Geometry check sheet. Reference: drawing and pictorial views, mm from the part's lowest x, y, z. A direction names the side the tool comes from. Round coordinates to 2 decimals unless told otherwise and drop trailing zeros. Write each loop counter-clockwise with the first axis right and the second up, starting at its lowest first coordinate (ties: lowest second). Pieces come first, ordered by that corner, then holes. Notation, with made-up numbers: (57.25, -2.5) -> (95.25, -2.5) arc R34 cw to (95.25, 30.5) -> close; hole circle Ø1 at (-16, -35.75). An arc over 180 degrees is marked (long way). Answer as a JSON object with one key per item and string values. Group by question number.
(1) Gauge pin test, flat ends, axial feed: pin 1 Ø4 at (x, z) = (964, 54) entering from -Y; pin 2 Ø8 at (x, y) = (710, 92.5) entering from +Z. Record the tip position at first contact, or that the pin passes through.
(2) Sectioned sample at A-A on z = 294.5. Record the cut outline in (x, y), and give its area (3 significant figures).
(3) Sectioned sample at B-B on x = 579. Record the cut outline in (y, z).
(4) Scan lines: L1, parallel to Y at x = 508, z = 308; L2, parallel to X at y = 81.5, z = 136.5. Record each from-to range of solid material in increasing order. Write a range as from..to.
(5) Sectioned sample at C-C on y = 43. Record the cut outline in (x, z), and give its area (3 significant figures).
(6) Set-up check for the marked faces 1 and 2: record each of +Z, -Z, +X, -X, +Y, -Y from which the full face is reachable in a straight line by a thin tool's end or side.
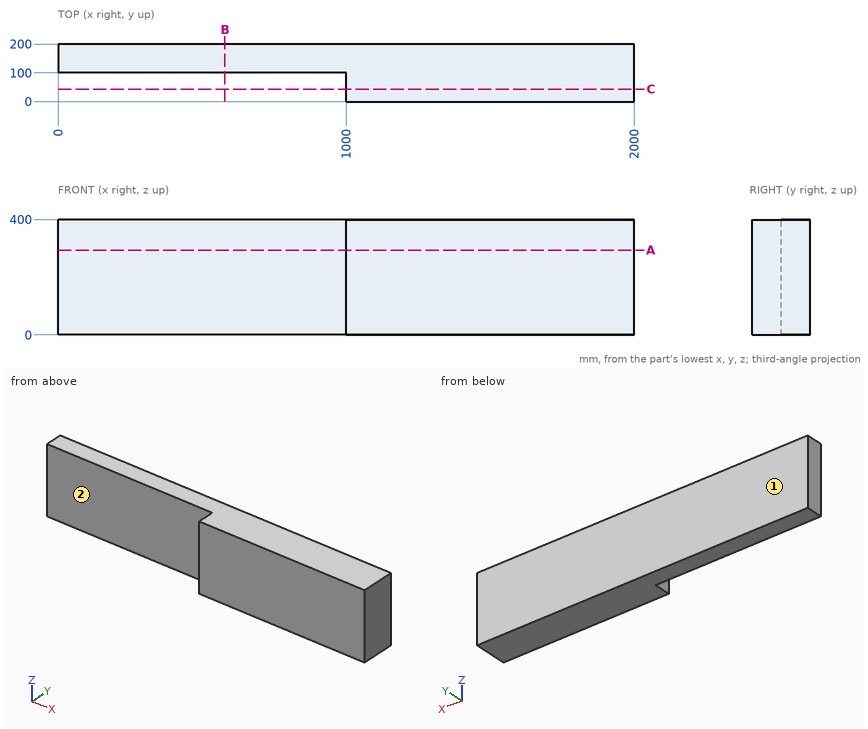
Computed values:
{
 "1": {"pin 1": "y = 100", "pin 2": "through"},
 "2": {"outline": "(0, 100) -> (1000, 100) -> (1000, 0) -> (2000, 0) -> (2000, 200) -> (0, 200) -> close", "area": "300,000 mm2"},
 "3": {"outline": "(100, 0) -> (200, 0) -> (200, 400) -> (100, 400) -> close"},
 "4": {"L1": "100..200", "L2": "1000..2000"},
 "5": {"outline": "(1000, 0) -> (2000, 0) -> (2000, 400) -> (1000, 400) -> close", "area": "400,000 mm2"},
 "6": {"face 1": "+Z, -Z, +X, -X, +Y", "face 2": "+Z, -Z, -X, -Y"}
}
